The listing builds one solid part. Answer for the finished solid, in the listing's coordinates (mm). Face numbers are marked on the shaded views. A direction names the side the tool comes from. Round coordinates to 2 decimals unless told otherwise and drop trailing zeros. Write each loop counter-clockwise with the first axis right and the second up, starting at its lowest first coordinate (ties: lowest second). Pieces come first, ordered by that corner, then holes.
(1) The mould has two halves that part along X. Classify the marked faces 1, 2, 3 and 4: +X half, -X half, draft (parallel to the pull), parting line (faces both ways), or undercut.
(2) Each of these flat-tipped pins is pushed along its axis until it touches: pin 1 Ø5 at (x, z) = (-25, 1.5) entering from +Y; pin 2 Ø4.5 at (x, z) = (-11, 1.5) entering from -Y; pin 3 Ø3 at (y, z) = (21.5, -1) entering from -X; pin 4 Ø3 at (x, z) = (-25, 0) entering from -Y. Where does it stop, or does it pass through?
(3) Find the intervals of material crossed by probe 1 along X at (y, z) = (-12, 2.25); probe 2 along Z at (x, y) = (-25, -23); probe 3 along X at (y, z) = (-25, 2.75), in increasing order.
(4) A cutting plane is placed at A-A, the plane y = -22. Give the vertices of the cut face in (x, z).
(5) A cutting plane is placed at D-D, the plane z = -3.75. Give the vertices of the cut face in (x, y).
(6) For the marked faces 5, 6 and 7, determine the directions among +Z, -Z, +X, -X, +Y, -Y from which every point of the face is accessible in a straight line to the end or side of a thin tool.
(7) A cutting plane is placed at B-B, the plane x = -25. Give the vertices of the cut face in (y, z).
(8) A cutting plane is placed at C-C, the plane y = 9.8. Give the vertices of the cut face in (x, z), and give its area (3 significant figures).
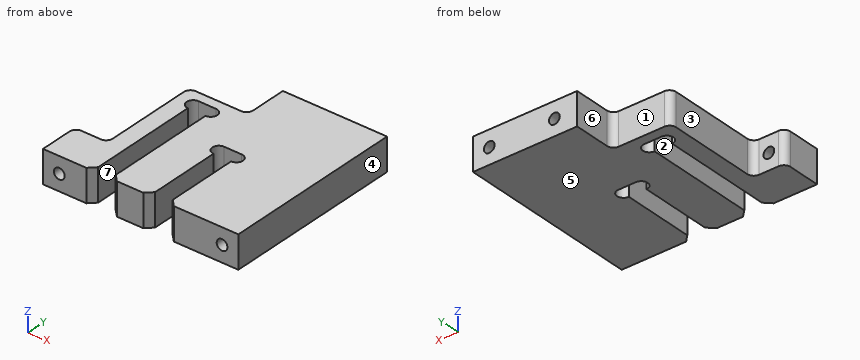
from build123d import *

# Parameters (mm, degrees)
SKETCH_1_W             = 60
SKETCH_1_H             = 56
EXTRUDE_1_DEPTH        = 5
SKETCH_3_W             = 5.4
SKETCH_3_H             = 28
SKETCH_3_H_2           = 39.8
CUT_EXTRUDE_1_DEPTH    = 43.237424164
HOLE_WIZARD_M4_1_D     = 3.3
HOLE_WIZARD_M4_1_DEPTH = 12.1
HOLE_WIZARD_M4_1_TIP   = 0.991420021
MM_1_D                 = 4
MM_1_DEPTH             = 13
MM_1_TIP               = 1.201721238
CHAMFER_1_SIZE         = 2
CUT_EXTRUDE_4_DEPTH    = 43.237424164
FILLET_2_R             = 2
HOLE_WIZARD_M4_2_D     = 3.3
HOLE_WIZARD_M4_2_DEPTH = 12.1
HOLE_WIZARD_M4_2_TIP   = 0.991420021


with BuildPart() as part:
    # 草图1 → 凸台-拉伸1 (new, symmetric)
    with BuildSketch(Plane.XY):
        Rectangle(SKETCH_1_W, SKETCH_1_H)
    extrude(amount=EXTRUDE_1_DEPTH, both=True)

    # 草图3 → 切除-拉伸1 (cut, through all)
    with BuildSketch(Plane.XY.offset(5)):
        with Locations((5.51, -14)):
            Rectangle(SKETCH_3_W, SKETCH_3_H)
        with Locations((-11.99, -8.1)):
            Rectangle(SKETCH_3_W, SKETCH_3_H_2)
    extrude(amount=-CUT_EXTRUDE_1_DEPTH, mode=Mode.SUBTRACT)

    # M4 螺纹孔1
    with Locations(Plane(origin=(0, -28, 0), x_dir=(-1, 0, 0), z_dir=(0, -1, 0))):
        with Locations((25, 0), (-25, 0)):
            Hole(HOLE_WIZARD_M4_1_D / 2, depth=HOLE_WIZARD_M4_1_DEPTH)
            with Locations((0, 0, -(HOLE_WIZARD_M4_1_DEPTH + HOLE_WIZARD_M4_1_TIP / 2))):  # 118° drill point
                Cone(0, HOLE_WIZARD_M4_1_D / 2, HOLE_WIZARD_M4_1_TIP, mode=Mode.SUBTRACT)

    # 大小mm 暗销孔1
    with Locations(Plane.XY.offset(5)):
        with Locations((-14.69, 9.8), (-9.29, 9.8), (2.81, -2), (8.21, -2)):
            Hole(MM_1_D / 2, depth=MM_1_DEPTH)
            with Locations((0, 0, -(MM_1_DEPTH + MM_1_TIP / 2))):  # 118° drill point
                Cone(0, MM_1_D / 2, MM_1_TIP, mode=Mode.SUBTRACT)

    # 倒角1
    chamfer_1_edges = [part.edges().sort_by_distance(p)[0] for p in [
        (2.81, -28, 0),
        (8.21, -28, 0),
        (-9.29, -28, 0),
        (-14.69, -28, 0),
    ]]
    chamfer(chamfer_1_edges, length=CHAMFER_1_SIZE)

    # 草图13 → 切除-拉伸4 (cut, through all)
    with BuildSketch(Plane.XY.offset(5)):
        Polygon((-30, 28), (-2, 28), (-2, 14.8), (-20, 14.8), (-20, -16), (-30, -16), align=None)
    extrude(amount=-CUT_EXTRUDE_4_DEPTH, mode=Mode.SUBTRACT)

    # 圆角2
    fillet_2_edges = [part.edges().sort_by_distance(p)[0] for p in [
        (-20, -16, 0),
        (-30, -16, 0),
        (-2, 14.8, 0),
        (-20, 14.8, 0),
    ]]
    fillet(fillet_2_edges, radius=FILLET_2_R)

    # M4 螺纹孔2
    with Locations(Plane(origin=(0, 28, 0), x_dir=(1, 0, 0), z_dir=(0, 1, 0))):
        with Locations((25, 0), (5, 0)):
            Hole(HOLE_WIZARD_M4_2_D / 2, depth=HOLE_WIZARD_M4_2_DEPTH)
            with Locations((0, 0, -(HOLE_WIZARD_M4_2_DEPTH + HOLE_WIZARD_M4_2_TIP / 2))):  # 118° drill point
                Cone(0, HOLE_WIZARD_M4_2_D / 2, HOLE_WIZARD_M4_2_TIP, mode=Mode.SUBTRACT)


solid = part.part
Solutions:
1. face 1: draft
1. face 2: undercut
1. face 3: -X half
1. face 4: +X half
2. pin 1: stops at y = -16
2. pin 2: stops at y = -26.54
2. pin 3: stops at x = -2
2. pin 4: passes through
3. probe 1: x = -20 to -14.69, -9.29 to 2.81, 8.21 to 30
3. probe 2: z = -5 to -1.65, 1.65 to 5
3. probe 3: x = -30 to -14.69, -9.29 to 2.81, 8.21 to 30
4. outline: (-30, -5) - (-14.69, -5) - (-14.69, 5) - (-30, 5) - close; (-9.29, -5) - (2.81, -5) - (2.81, 5) - (-9.29, 5) - close; (8.21, -5) - (30, -5) - (30, 5) - (8.21, 5) - close; hole circle Ø3.3 at (-25, 0); hole circle Ø3.3 at (25, 0)
5. outline: (-30, -28) - (-16.69, -28) - (-14.69, -26) - (-14.69, 7.8) arc R2 cw to (-14.69, 11.8) - (-9.29, 11.8) arc R2 cw to (-9.29, 7.8) - (-9.29, -26) - (-7.29, -28) - (0.81, -28) - (2.81, -26) - (2.81, -4) arc R2 cw to (2.81, 0) - (8.21, 0) arc R2 cw to (8.21, -4) - (8.21, -26) - (10.21, -28) - (30, -28) - (30, 28) - (-2, 28) - (-2, 16.8) arc R2 cw to (-4, 14.8) - (-18, 14.8) arc R2 ccw to (-20, 12.8) - (-20, -14) arc R2 cw to (-22, -16) - (-28, -16) arc R2 ccw to (-30, -18) - close
6. face 5: -Z, +X, -X, +Y, -Y
6. face 6: +Z, -Z, -X, +Y
6. face 7: +Z, -Z, -Y
7. outline: (-28, -5) - (-16, -5) - (-16, -1.65) - (-28, -1.65) - close; (-28, 1.65) - (-16, 1.65) - (-16, 5) - (-28, 5) - close
8. outline: (-20, -5) - (-16.69, -5) - (-16.69, 5) - (-20, 5) - close; (-7.29, -5) - (30, -5) - (30, 5) - (-7.29, 5) - close
8. area: 406 mm2
